Input: part model. Units: mm. Frame: model coordinates. A direction names the side the tool comes from. Coordinates: 2 decimals unless noted, no trailing zeros. Loops run counter-clockwise (first coordinate to the right, second up) from the corner with the lowest first, then second, coordinate; pieces in that order, holes last. Notation, with made-up numbers: M 8,10.5 L 27,10.5 A9 ccw 27,26.5 Z; hole C 18,63 d8. An arc over 180 degrees is marked long. Use a Markdown table: item, result. Add a question column.
1. Set-up query: faces 1 (the flat face through (2, 0, 1)), 2 (the flat face through (3, -5, 3)). Return all of +Z, -Z, +X, -X, +Y, -Y with unobstructed straight access to the full face (end or side cutting, diameter ignored); none if empty.
2. Section A-A on x = 0. Output: boundary loops of the cut face in (y, z).
3. Section B-B on z = 2.1. Output: boundary loops of the cut face in (x, y), then the cut area to 3 significant figures.
4. Line query: L1, parallel to Y at x = 0, z = 1.55; L2, parallel to X at y = 0.5, z = 1.4; L3, parallel to Z at x = -2.5, y = 2.5. Output: solid intervals per line, ascending. Write a range as [from, to].
5. Section C-C on z = 0.7. Output: boundary loops of the cut face in (x, y), then the cut area to 3 significant figures.
6. Draft query along Y for faces 3 (the cylindrical face through (-1.73, -7.81, 1.23)), 4 (the flat face through (1.05, 0, 0.5)), 5 (the flat face through (2, 0, 0)). Return one class per face: +Y half, -Y half, draft (parallel to the pull), parting line (faces both ways), or undercut.
7. Pin query (flat end, axial travel): pin 1 (3 mm diameter, centred on x = 1, y = 0.5, fed in from +Z); pin 2 (0.5 mm diameter, centred on y = 0.5, z = 0.5, fed in from -X). Return the tip coordinate at first contact, or that it passes through.
```python
from build123d import *

# Parameters (mm, degrees)
F0_R     = 5.3
F1_DEPTH = 1
F0_R_2   = 8
F2_DEPTH = 3
F3_R     = 0.5


with BuildPart() as f1:
    # F0 (on Top) → F1 (new body)
    with BuildSketch(Plane.XY):
        Circle(F0_R)
        with BuildLine():
            ThreePointArc((1.05, 1.4), (1.5652475842, 0.7826237921), (1.75, 0))
            ThreePointArc((1.75, 0), (1.5652475842, -0.7826237921), (1.05, -1.4))
            ThreePointArc((1.05, -1.4), (-0.7826237921, -1.5652475842), (-1.75, 0))
            ThreePointArc((-1.75, 0), (-0.7826237921, 1.5652475842), (1.05, 1.4))
        make_face(mode=Mode.SUBTRACT)
        with BuildLine():
            ThreePointArc((1.05, -1.4), (1.5652475842, -0.7826237921), (1.75, 0))
            ThreePointArc((1.75, 0), (1.5652475842, 0.7826237921), (1.05, 1.4))
            Line((1.05, 1.4), (1.05, 0))
            Line((1.05, 0), (1.05, -1.4))
        make_face()
    extrude(amount=F1_DEPTH)

    # F0 (on Top) → F2 (join)
    with BuildSketch(Plane.XY):
        Circle(F0_R_2)
        Circle(F0_R, mode=Mode.SUBTRACT)
    extrude(amount=F2_DEPTH)

    # F3
    f3_edges = [f1.edges().sort_by_distance(p)[0] for p in [
        (-8, 0, 3),
    ]]
    fillet(f3_edges, radius=F3_R)


solid = f1.part
```
Answers below:
| question | item | result |
|---|---|---|
| 1 | face 1 | +Z |
| 1 | face 2 | +Z, +X, -X, +Y, -Y |
| 2 | outline | M -8,0 L -1.75,0 L -1.75,1 L -5.3,1 L -5.3,3 L -7.5,3 A0.5 ccw -8,2.5 Z; M 1.75,0 L 8,0 L 8,2.5 A0.5 ccw 7.5,3 L 5.3,3 L 5.3,1 L 1.75,1 Z |
| 3 | outline | C 0,0 d16; hole C 0,0 d10.6 |
| 3 | area | 113 mm² |
| 4 | L1 | y = [-8, -5.3], [5.3, 8] |
| 4 | L2 | x = [-7.98, -5.28], [5.28, 7.98] |
| 4 | L3 | z = [0, 1] |
| 5 | outline | C 0,0 d16; hole M 1.05,-1.4 L 1.05,1.4 A1.75 ccw long Z |
| 5 | area | 193 mm² |
| 6 | face 3 | parting line |
| 6 | face 4 | undercut |
| 6 | face 5 | draft |
| 7 | pin 1 | stops at z = 1 |
| 7 | pin 2 | stops at x = -8 |
